```python
from build123d import *

# Parameters (mm, degrees)
SKETCH_1_R          = 1.8
SKETCH_1_R_2        = 12
EXTRUDE_1_DEPTH     = 5
SKETCH_4_W          = 42
SKETCH_4_H          = 4
EXTRUDE_2_DEPTH     = 27
SKETCH_5_R          = 2.25
CUT_EXTRUDE_1_DEPTH = 4
CHAMFER_1_SIZE      = 3
EXTRUDE_3_DEPTH     = 3
CHAMFER_2_SIZE      = 3


with BuildPart() as part:
    # 草图1 → 凸台-拉伸1 (new body)
    with BuildSketch(Plane.XY):
        Polygon((-21, 21), (-21, -21), (21, -21), (21, 21), (21, 50), (-21, 50), align=None)
        with Locations((-15.5, -16)):
            Circle(SKETCH_1_R, mode=Mode.SUBTRACT)
        with Locations((-15.5, 15)):
            Circle(SKETCH_1_R, mode=Mode.SUBTRACT)
        with Locations(Location((15.5, -16, 0), (0, 0, 180))):
            Circle(SKETCH_1_R, mode=Mode.SUBTRACT)
        with Locations(Location((15.5, 15, 0), (0, 0, 180))):
            Circle(SKETCH_1_R, mode=Mode.SUBTRACT)
        Circle(SKETCH_1_R_2, mode=Mode.SUBTRACT)
    extrude(amount=EXTRUDE_1_DEPTH)

    # 草图4 → 凸台-拉伸2 (add)
    with BuildSketch(Plane.XY.offset(5)):
        with Locations((0, 48)):
            Rectangle(SKETCH_4_W, SKETCH_4_H)
    extrude(amount=EXTRUDE_2_DEPTH)

    # 草图5 → 切除-拉伸1 (cut)
    with BuildSketch(Plane(origin=(0, 50, 0), x_dir=(1, 0, 0), z_dir=(0, 1, 0))):
        with Locations(Location((-16, -27, 0), (0, 0, 270))):
            Circle(SKETCH_5_R)
        with Locations(Location((-8, -27, 0), (0, 0, 270))):
            Circle(SKETCH_5_R)
        with Locations(Location((0, -27, 0), (0, 0, 270))):
            Circle(SKETCH_5_R)
        with Locations(Location((8, -27, 0), (0, 0, 270))):
            Circle(SKETCH_5_R)
        with Locations(Location((16, -27, 0), (0, 0, 270))):
            Circle(SKETCH_5_R)
        with Locations(Location((-16, -19, 0), (0, 0, 270))):
            Circle(SKETCH_5_R)
        with Locations(Location((-8, -19, 0), (0, 0, 270))):
            Circle(SKETCH_5_R)
        with Locations(Location((0, -19, 0), (0, 0, 270))):
            Circle(SKETCH_5_R)
        with Locations(Location((8, -19, 0), (0, 0, 270))):
            Circle(SKETCH_5_R)
        with Locations(Location((16, -19, 0), (0, 0, 270))):
            Circle(SKETCH_5_R)
        with Locations(Location((-16, -11, 0), (0, 0, 270))):
            Circle(SKETCH_5_R)
        with Locations(Location((-8, -11, 0), (0, 0, 270))):
            Circle(SKETCH_5_R)
        with Locations(Location((0, -11, 0), (0, 0, 270))):
            Circle(SKETCH_5_R)
        with Locations(Location((8, -11, 0), (0, 0, 270))):
            Circle(SKETCH_5_R)
        with Locations(Location((16, -11, 0), (0, 0, 270))):
            Circle(SKETCH_5_R)
    extrude(amount=-CUT_EXTRUDE_1_DEPTH, mode=Mode.SUBTRACT)

    # 倒角1
    chamfer_1_edges = [part.edges().sort_by_distance(p)[0] for p in [
        (21, -21, 2.5),
        (-21, -21, 2.5),
        (21, 48, 32),
        (-21, 48, 32),
    ]]
    chamfer(chamfer_1_edges, length=CHAMFER_1_SIZE)

    # 草图7 → 凸台-拉伸3 (add)
    with BuildSketch(Plane.ZY.offset(21)):
        Polygon((29, 46), (5, 22), (0, 22), (0, 50), (29, 50), align=None)
    extrude_3 = extrude(amount=EXTRUDE_3_DEPTH)

    # 镜向1: 凸台-拉伸3 across plane
    add(extrude_3.mirror(Plane(origin=(0, 0, 0), x_dir=(0, 0, 1), z_dir=(1, 0, 0))))

    # 倒角2
    chamfer_2_edges = [part.edges().sort_by_distance(p)[0] for p in [
        (24, 22, 2.5),
        (24, 48, 29),
        (-24, 48, 29),
        (-24, 22, 2.5),
    ]]
    chamfer(chamfer_2_edges, length=CHAMFER_2_SIZE - 0.0001)  # a hair under: the kernel refuses the full size


solid = part.part
```
For this review, take the finished solid that the model builds, in its own axes (mm). A direction names the side the tool comes from. Give positions to 0.01 mm unless a question says otherwise; leave off trailing zeros. Order: outer loops, then holes, each group sorted by start corner. A loop starts at its lowest first (then second) coordinate and runs counter-clockwise, first axis right, second up.
1) The part is to be moulded in two halves that separate along Z. For faces 1 (the face through (0, 46, 15)), 2 (the face through (9.52, 48.03, 9.34)), 3 (the face through (-19, 48, 31)), say which applies: released by +Z, released by -Z, zero draft, split by the parting line, or undercut.
2) Take a section at C-C (y = 35). Give the boundary of the cut face in (x, z).
3) Insertion check: pin 1 (7 mm diameter, centred on x = 8, z = 11, fed in from -Y); pin 2 (5 mm diameter, centred on x = -8, z = 10.5, fed in from +Y); pin 3 (2.5 mm diameter, centred on y = 6.5, z = 2, fed in from -X); pin 4 (12.5 mm diameter, centred on x = 1, y = 6.5, fed in from +Z). Each pin has a flat end and moves straight along its axis. Give the tip position at first contact, or say it passes through.
4) Take a section at B-B (x = 0). Give the boundary of the cut face in (y, z), then the cut area to 3 significant figures.
5) Wall thickness on line 1 (X direction, y = 49.1, z = 11); line 2 (Y direction, x = 0, z = 3.15); line 3 (Z direction, x = 13, y = -8.5): over which ranges is each line inside the solid? List them lowest first.
6) Take a section at A-A (y = 15). Give the boundary of the cut face in (x, z), then the cut area to 3 significant figures.
7) For faces 4 (the face through (21, 2, 2)), 5 (the face through (21, 40, 12)), 6 (the face through (14.004, 48.028, 28.038)), list the 3-axis set-ups (+Z, -Z, +X, -X, +Y, -Y) from which the entire face can be reached by the end or side of a thin tool; tool diameter is ignored.
8) Take a section at D-D (z = 27). Give the boundary of the cut face in (x, y).
Derived:
1. face 1: zero draft
1. face 2: undercut
1. face 3: released by +Z
2. outline: (-24, 0) - (24, 0) - (24, 18) - (21, 18) - (21, 5) - (-21, 5) - (-21, 18) - (-24, 18) - close
3. pin 1: stops at y = 46
3. pin 2: stops at y = 50
3. pin 3: stops at x = -21
3. pin 4: stops at z = 5
4. outline: (-21, 0) - (-12, 0) - (-12, 5) - (-21, 5) - close; (12, 0) - (50, 0) - (50, 8.75) - (46, 8.75) - (46, 5) - (12, 5) - close; (46, 13.25) - (50, 13.25) - (50, 16.75) - (46, 16.75) - close; (46, 21.25) - (50, 21.25) - (50, 24.75) - (46, 24.75) - close; (46, 29.25) - (50, 29.25) - (50, 32) - (46, 32) - close
4. area: 289 mm2
5. line 1: x = -24 to -18.25, -13.75 to -10.25, -5.75 to -2.25, 2.25 to 5.75, 10.25 to 13.75, 18.25 to 24
5. line 2: y = -21 to -12, 12 to 50
5. line 3: z = 0 to 5
6. outline: (-21, 0) - (-17.3, 0) - (-17.3, 5) - (-21, 5) - close; (-13.7, 0) - (13.7, 0) - (13.7, 5) - (-13.7, 5) - close; (17.3, 0) - (21, 0) - (21, 5) - (17.3, 5) - close
6. area: 174 mm2
7. face 4: +Z, -Z, +X, -Y
7. face 5: +Z, -Y
7. face 6: +Y, -Y
8. outline: (-23, 44) - (-21, 44) - (-21, 46) - (-18.25, 46) - (-18.25, 50) - (-23, 50) - close; (-13.75, 46) - (-10.25, 46) - (-10.25, 50) - (-13.75, 50) - close; (-5.75, 46) - (-2.25, 46) - (-2.25, 50) - (-5.75, 50) - close; (2.25, 46) - (5.75, 46) - (5.75, 50) - (2.25, 50) - close; (10.25, 46) - (13.75, 46) - (13.75, 50) - (10.25, 50) - close; (18.25, 46) - (21, 46) - (21, 44) - (23, 44) - (23, 50) - (18.25, 50) - close
